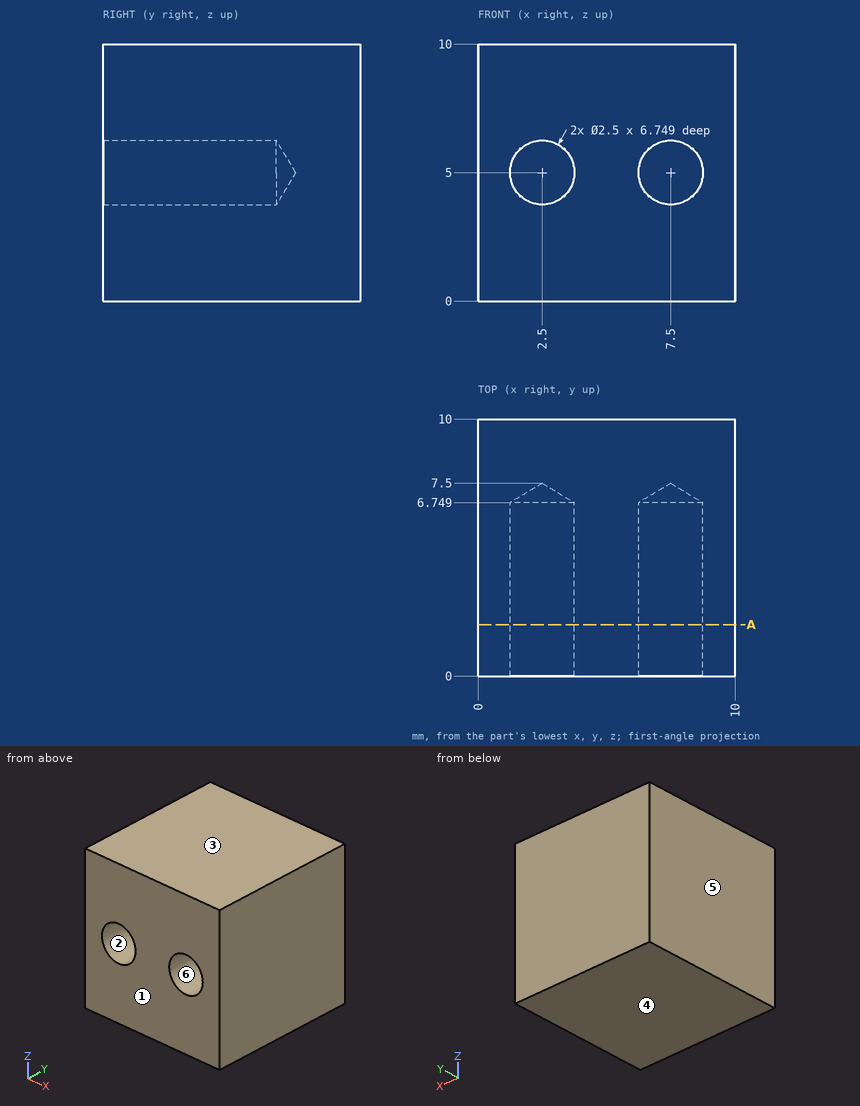
Verification items for this drawing (mm, ordinates from the low corner). A direction names the side the tool comes from. Give positions to 0.01 mm unless a question says otherwise; leave off trailing zeros. Loops run counter-clockwise (first coordinate to the right, second up) from the corner with the lowest first, then second, coordinate; pieces in that order, holes last. Notation, with made-up numbers: M -1,27 L 35,27 A5 cw 35,33 Z; hole C 21,83.5 d2. An arc over 180 degrees is marked long. Write each question's results on one line, items separated by ' | '.
1) Thickness scan on line 1 (X direction, y = 5.75, z = 5); line 2 (Z direction, x = 7.5, y = 4.75); line 3 (Z direction, x = 3.25, y = 3). Record the ranges inside material, lowest first.
Answers follow:
line 1: 0 to 1.25, 3.75 to 6.25, 8.75 to 10 | line 2: 0 to 3.75, 6.25 to 10 | line 3: 0 to 4, 6 to 10
2) Section check A-A, the plane y = 2. Record the boundary of the cut face in (x, z).
Answers follow:
outline: M 0,0 L 10,0 L 10,10 L 0,10 Z; hole C 2.5,5 d2.5; hole C 7.5,5 d2.5
3) Release check for a two-part mould opening along Z. For the marked faces 1, 2, 3 and 4 record: +Z half, -Z half, draft (parallel to the pull), parting line (faces both ways), or undercut.
Answers follow:
face 1: draft | face 2: undercut | face 3: +Z half | face 4: -Z half
4) Gauge pin test, flat end, axial feed: pin 1 (2 mm diameter, centred on x = 7.5, z = 5, fed in from -Y). Record the tip position at first contact, or that the pin passes through.
Answers follow:
pin 1: y = 6.9
5) Tool access check on the marked faces 5 and 6. Record the directions out of +Z, -Z, +X, -X, +Y, -Y that give a thin tool (end or side, any length) a straight path to the whole face; none if there is none.
Answers follow:
face 5: +Z, -Z, -X, +Y, -Y | face 6: -Y
